```python
from build123d import *

# Parameters (mm, degrees)
BOSS_EXTRUDE2_DEPTH = 482.6


with BuildPart() as part:
    # Sketch2 → Boss-Extrude2 (new body)
    with BuildSketch(Plane(origin=(0, 0, 0), x_dir=(0, 0, -1), z_dir=(1, 0, 0))):
        with BuildLine():
            Line((0, 0), (0, 54.346487563))
            Line((0, 54.346487563), (3.96875, 54.346487563))
            Line((3.96875, 54.346487563), (3.96875, 11.151453071))
            ThreePointArc((3.96875, 11.151453071), (21.455972099, 8.967240909), (38.1, 3.175))
            Line((38.1, 3.175), (38.1, 0))
            Line((38.1, 0), (0, 0))
        make_face()
    boss_extrude2 = extrude(amount=-BOSS_EXTRUDE2_DEPTH)

    # Mirror1: Boss-Extrude2 across plane
    add(boss_extrude2.mirror(Plane(origin=(-482.6, 0, 0), x_dir=(1, 0, 0), z_dir=(0, 0, 1))))


solid = part.part
```
Part model, mm, in its own coordinate system. A direction names the side the tool comes from. Round coordinates to 2 decimals unless told otherwise and drop trailing zeros. Order: outer loops, then holes, each group sorted by start corner. A loop starts at its lowest first (then second) coordinate and runs counter-clockwise, first axis right, second up. Notation, with made-up numbers: M -1,39.5 L 56,39.5 A17 cw 56,67.5 Z; hole C 19.25,86 d4. An arc over 180 degrees is marked long. Put each result on its own line as item: value. Start each with the question number.
1. Tool access for faces 1 (the face through (-482.6, 13, 0)), 2 (the face through (-238, 33, -3.969)), 3 (the face through (-238, 33, 3.969)): list every direction of +Z, -Z, +X, -X, +Y, -Y with a clear straight run to the whole face (end or side of a thin tool).
2. Slice it at B-B on y = 25.5. List the corners of the cut face in (x, z).
3. Drill centre lines: probe 1 along Z at (x, y) = (-413, 28); probe 2 along Y at (x, z) = (-151, -4); probe 3 along Y at (x, z) = (-245, -32). Where is each one in solid material? Low to high. Write a range as [from, to].
4. Slice it at A-A on x = -68. List the corners of the cut face in (y, z) (3 decimals).
5. Drop flat-ended pins along their axis: pin 1 (12 mm diameter, centred on x = -195, y = 33.5, fed in from +Z); pin 2 (6 mm diameter, centred on x = -232.5, z = 17, fed in from +Y); pin 3 (13 mm diameter, centred on x = -309.5, y = 36, fed in from -Z). Give the stop position or say it passes through.
6. Slice it at C-C on z = -29. List the corners of the cut face in (x, y), then the cut area to 3 significant figures.
Findings:
1. face 1: +Z, -Z, -X, +Y, -Y
1. face 2: -Z, +X, -X, +Y
1. face 3: +Z, +X, -X, +Y
2. outline: M -482.6,-3.97 L 0,-3.97 L 0,3.97 L -482.6,3.97 Z
3. probe 1: [-3.97, 3.97]
3. probe 2: [0, 11.15]
3. probe 3: [0, 5.76]
4. outline: M 0,-38.1 L 3.175,-38.1 A83.82 ccw 11.151,-3.969 L 54.346,-3.969 L 54.346,3.969 L 11.151,3.969 A83.82 ccw 3.175,38.1 L 0,38.1 Z
5. pin 1: z = 3.97
5. pin 2: y = 10.36
5. pin 3: z = -3.97
6. outline: M -482.6,0 L 0,0 L 0,6.83 L -482.6,6.83 Z
6. area: 3,290 mm2
